from build123d import *

# Parameters (mm, degrees)
EXTRUDE_1_DEPTH     = 530
SKETCH_2_OUTSIDE_W  = 646.648
SKETCH_2_OUTSIDE_H  = 155.148
CUT_EXTRUDE_2_DEPTH = 216
SKETCH_3_R          = 5
SKETCH_3_R_2        = 66
CUT_EXTRUDE_3_DEPTH = 3


with BuildPart() as part:
    # Эскиз1 → Вытянуть-Тонкостенный1 (new body)
    with BuildSketch(Plane(origin=(0, 0, 0), x_dir=(0, 0, -1), z_dir=(1, 0, 0))):
        Polygon((-105, 38.5), (-105, 0), (110, 0), (110, 38.5), (108, 38.5), (108, 2), (-103, 2), (-103, 38.5), align=None)
    extrude(amount=EXTRUDE_1_DEPTH)

    # Эскиз2 outside → Вырез-Вытянуть2 (cut, through all)
    with BuildSketch(Plane(origin=(0, 0, -110), x_dir=(-1, 0, 0), z_dir=(0, 0, -1))):
        with Locations((-265, 19.25)):
            Rectangle(SKETCH_2_OUTSIDE_W, SKETCH_2_OUTSIDE_H)
        Polygon((-530, 0), (-530, 3), (-375, 38.5), (-155, 38.5), (0, 3), (0, 0), align=None, mode=Mode.SUBTRACT)
    extrude(amount=-CUT_EXTRUDE_2_DEPTH, mode=Mode.SUBTRACT)

    # Эскиз3 → Вырез-Вытянуть3 (cut, through all)
    with BuildSketch(Plane(origin=(0, 2, 0), x_dir=(1, 0, 0), z_dir=(0, 1, 0))):
        with Locations((20, 80)):
            Circle(SKETCH_3_R)
        with Locations((20, -75)):
            Circle(SKETCH_3_R)
        with Locations((510, 80)):
            Circle(SKETCH_3_R)
        with Locations((510, -75)):
            Circle(SKETCH_3_R)
        with Locations((265, 2.5)):
            Circle(SKETCH_3_R_2)
        with Locations((323.513972874, 61.013972874)):
            Circle(SKETCH_3_R)
        with Locations((323.513972874, -56.013972874)):
            Circle(SKETCH_3_R)
        with Locations((206.486027126, -56.013972874)):
            Circle(SKETCH_3_R)
        with Locations((206.486027126, 61.013972874)):
            Circle(SKETCH_3_R)
    extrude(amount=-CUT_EXTRUDE_3_DEPTH, mode=Mode.SUBTRACT)


solid = part.part
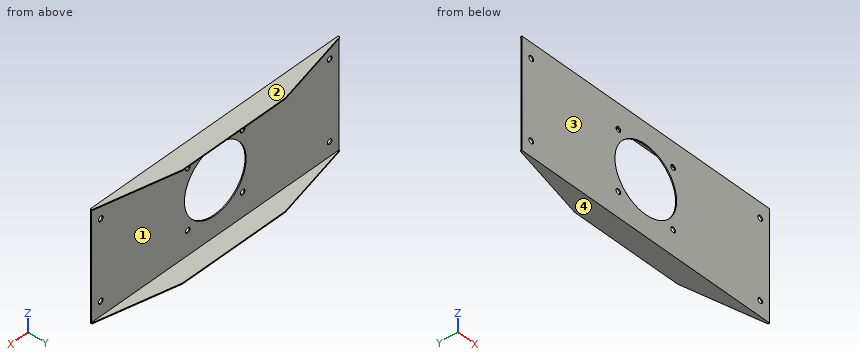
Can you work these out from the model? Positions are in its coordinate system, mm. Face numbers are marked on the shaded views. Coordinates: 2 decimals unless noted, no trailing zeros. Order: outer loops, then holes, each group sorted by start corner. A loop starts at its lowest first (then second) coordinate and runs counter-clockwise, first axis right, second up. Notation, with made-up numbers: (25, 7.25) - (72, 7.25) arc R15 ccw to (72, 15.25) - close; hole circle Ø7 at (21.5, -16). An arc over 180 degrees is marked (long way). Answer as a JSON object with one key per item and string values. Group by question number.
Q1. Imagine slicing it at A-A (x = 265). Please give me the cut outline in (y, z), and give its area (3 significant figures).
Q2. I need wall thicknesses on line 1 (X direction, y = 1.25, z = 75); line 2 (Z direction, x = 20, y = 0.65); line 3 (Z direction, x = 193.5, y = 28). Which ranges of each line are inside material? Lowest first, please. Write a range as from..to.
Q3. Will this pin go through, and if not, where does the flat tip stop? P1, Ø16, axis at x = 206.49, z = 56.01, coming from the +Y side.
Q4. We'd pull the mould along Z, two halves only. Please class the marked faces 1, 2, 3 and 4: +Z half, -Z half, draft (parallel to the pull), parting line (faces both ways), or undercut.
Q5. Imagine slicing it at B-B (z = -80). Please give me the cut outline in (x, y), and give its area (3 significant figures).
Q6. Imagine slicing it at C-C (y = 30.5). Please give me the cut outline in (x, z), and give its area (3 significant figures).
Q7. Imagine slicing it at D-D (x = 20). Please give me the cut outline in (y, z), and give its area (3 significant figures).
Determined:
{
 "1": {"outline": "(0, -110) - (38.5, -110) - (38.5, -108) - (2, -108) - (2, -68.5) - (0, -68.5) - close; (0, 63.5) - (2, 63.5) - (2, 103) - (38.5, 103) - (38.5, 105) - (0, 105) - close", "area": "312 mm2"},
 "2": {"line 1": "x = 0..15, 25..505, 515..530", "line 2": "z = -110..-85, -75..70, 80..105", "line 3": "z = -110..-108, 103..105"},
 "3": {"P1": "stops at y = 2"},
 "4": {"face 1": "undercut", "face 2": "+Z half", "face 3": "draft", "face 4": "-Z half"},
 "5": {"outline": "(0, 0) - (15, 0) - (15, 2) - (0, 2) - close; (25, 0) - (505, 0) - (505, 2) - (25, 2) - close; (515, 0) - (530, 0) - (530, 2) - (515, 2) - close", "area": "1,020 mm2"},
 "6": {"outline": "(120.07, -110) - (409.93, -110) - (409.93, -108) - (120.07, -108) - close; (120.07, 103) - (409.93, 103) - (409.93, 105) - (120.07, 105) - close", "area": "1,160 mm2"},
 "7": {"outline": "(0, -110) - (7.58, -110) - (7.58, -108) - (2, -108) - (2, -85) - (0, -85) - close; (0, -75) - (2, -75) - (2, 70) - (0, 70) - close; (0, 80) - (2, 80) - (2, 103) - (7.58, 103) - (7.58, 105) - (0, 105) - close", "area": "412 mm2"}
}
